Design review of the part shown in the three views and the two pictorial views. Dimensions are in mm from the part's minimum x, y and z. A direction names the side the tool comes from. Coordinates: 2 decimals unless noted, no trailing zeros. Write each loop counter-clockwise with the first axis right and the second up, starting at its lowest first coordinate (ties: lowest second). Pieces come first, ordered by that corner, then holes. Notation, with made-up numbers: (41.25, -28) -> (81.25, -28) arc R11 ccw to (81.25, -13) -> close; hole circle Ø8 at (70.5, 77). An arc over 180 degrees is marked (long way). Answer in a Markdown table with one row per item. Add a question column.
Item 1: To check wall thickness, follow line 1 (X direction, y = 1.5, z = 32.5); line 2 (Z direction, x = 4.75, y = 5); line 3 (Z direction, x = 2.5, y = 3.75). State the ranges of each line that lie inside material, in increasing order.
Item 2: Draft analysis for pull direction Y (two halves, no side actions). For the marked faces 1, 2 and 3, state which applies: released by +Y, released by -Y, zero draft, split by the parting line, or undercut.
Item 3: Take a section at A-A, the plane x = 4. Write out the cut boundary in (y, z).
Item 4: Clearance check with flat-ended pins moving along their axes: P1, Ø3.5, axis at y = 7, z = 28.5, coming from the +X side; P2, Ø1.5, axis at x = 5, z = 18, coming from the +Y side; P3, Ø3.5, axis at x = 11, y = 2, coming from the -Z side; P4, Ø2.5, axis at x = 6, y = 7, coming from the +Z side. State where each tip first meets the part, or that it passes through.
Item 5: Take a section at B-B, the plane y = 5.5. Write out the cut boundary in (x, z) (1 decimal).
Item 6: Take a section at D-D, the plane y = 8. Write out the cut boundary in (x, z) (1 decimal).
Item 7: Take a section at C-C, the plane z = 30. Write out the cut boundary in (x, y).
Item 8: For the marked faces 4, 5 and 6, list the 3-axis set-ups (+Z, -Z, +X, -X, +Y, -Y) from which the entire face can be reached by the end or side of a thin tool; tool diameter is ignored.
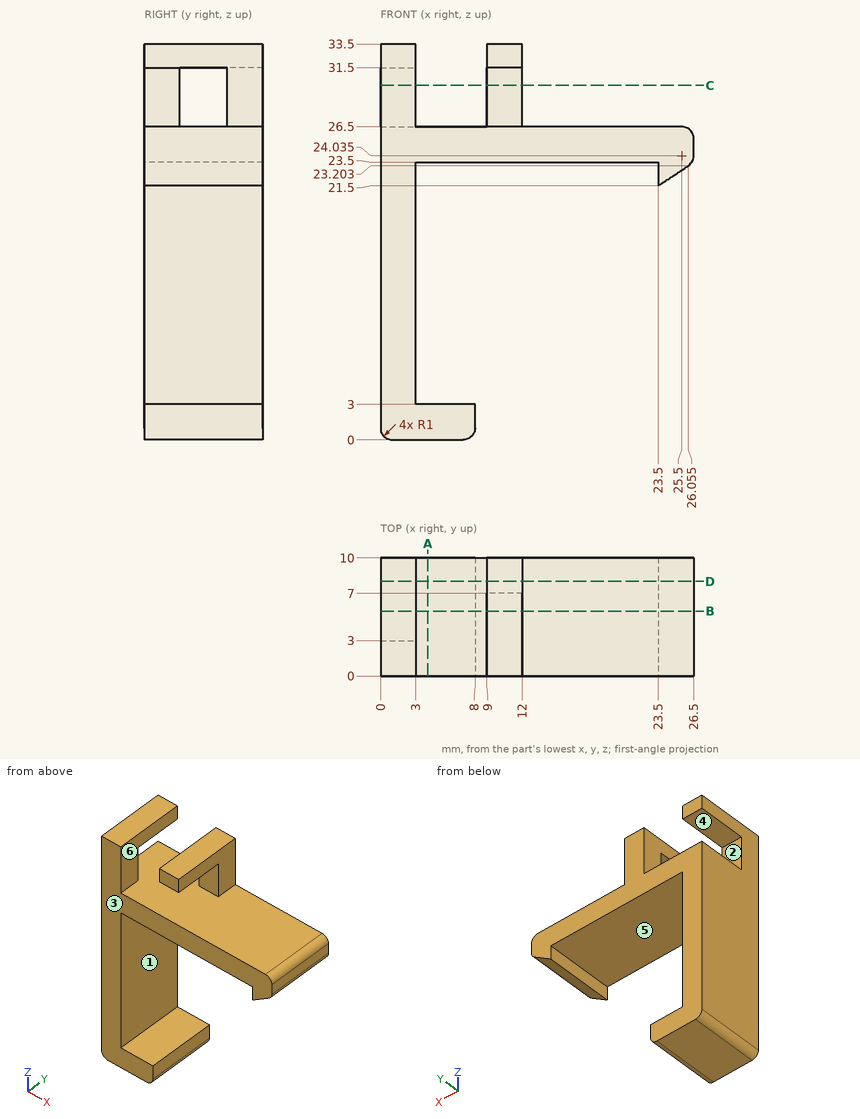
Answers:
| question | item | result |
|---|---|---|
| 1 | line 1 | x = 0 to 3, 9 to 12 |
| 1 | line 2 | z = 0 to 3, 23.5 to 26.5 |
| 1 | line 3 | z = 0 to 26.5, 31.5 to 33.5 |
| 2 | face 1 | zero draft |
| 2 | face 2 | released by +Y |
| 2 | face 3 | released by -Y |
| 3 | outline | (0, 0) -> (10, 0) -> (10, 3) -> (0, 3) -> close; (0, 23.5) -> (10, 23.5) -> (10, 26.5) -> (0, 26.5) -> close |
| 4 | P1 | stops at x = 12 |
| 4 | P2 | passes through |
| 4 | P3 | stops at z = 23.5 |
| 4 | P4 | stops at z = 26.5 |
| 5 | outline | (0, 1) arc R1 ccw to (1, 0) -> (7, 0) arc R1 ccw to (8, 1) -> (8, 3) -> (3, 3) -> (3, 23.5) -> (23.5, 23.5) -> (23.5, 21.5) -> (26.1, 23.2) arc R1 ccw to (26.5, 24) -> (26.5, 25.5) arc R1 ccw to (25.5, 26.5) -> (0, 26.5) -> close; (0, 31.5) -> (3, 31.5) -> (3, 33.5) -> (0, 33.5) -> close; (9, 31.5) -> (12, 31.5) -> (12, 33.5) -> (9, 33.5) -> close |
| 6 | outline | (0, 1) arc R1 ccw to (1, 0) -> (7, 0) arc R1 ccw to (8, 1) -> (8, 3) -> (3, 3) -> (3, 23.5) -> (23.5, 23.5) -> (23.5, 21.5) -> (26.1, 23.2) arc R1 ccw to (26.5, 24) -> (26.5, 25.5) arc R1 ccw to (25.5, 26.5) -> (12, 26.5) -> (12, 33.5) -> (9, 33.5) -> (9, 26.5) -> (0, 26.5) -> close; (0, 31.5) -> (3, 31.5) -> (3, 33.5) -> (0, 33.5) -> close |
| 7 | outline | (0, 0) -> (3, 0) -> (3, 3) -> (0, 3) -> close; (9, 7) -> (12, 7) -> (12, 10) -> (9, 10) -> close |
| 8 | face 4 | -X, +Y |
| 8 | face 5 | +Y, -Y |
| 8 | face 6 | +Z, +Y, -Y |
